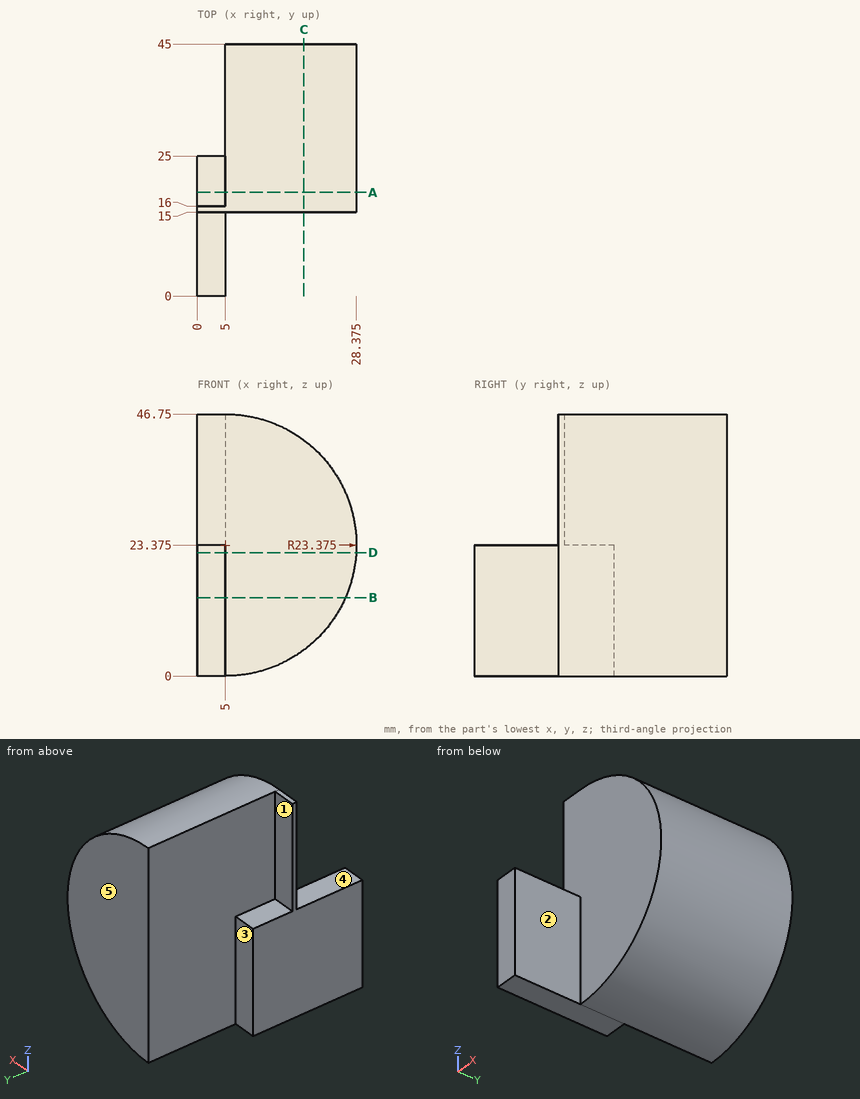
Design review of the part shown in the three views and the two pictorial views. Dimensions are in mm from the part's minimum x, y and z. A direction names the side the tool comes from. Round coordinates to 2 decimals unless told otherwise and drop trailing zeros. Loops run counter-clockwise (first coordinate to the right, second up) from the corner with the lowest first, then second, coordinate; pieces in that order, holes last.
1) Tool access review of the marked faces 1, 2, 3, 4 and 5: name each direction out of +Z, -Z, +X, -X, +Y, -Y from which nothing blocks a thin tool from reaching the whole face with its end or side.
Values follow:
face 1: +Z, -X, +Y
face 2: +Z, -Z, +X, -Y
face 3: +Z, -Z, -X, +Y
face 4: +Z, +X, -X, -Y
face 5: +Z, -Z, +X, -X, +Y
2) Consider section D-D on z = 22. State the section outline as (x, y) points, then the cut area to 3 significant figures.
Values follow:
outline: (0, 0) - (5, 0) - (5, 15) - (28.33, 15) - (28.33, 45) - (5, 45) - (5, 25) - (0, 25) - close
area: 825 mm2
3) Wall thickness on line 1 along Y through (x, z) = (24.25, 22.5); line 2 along X through (y, z) = (12, 20); line 3 along X through (y, z) = (27, 23): over which ranges is each line inside the solid? List them lowest first.
Values follow:
line 1: y = 15 to 45
line 2: x = 0 to 5
line 3: x = 5 to 28.37
4) Clearance check with flat-ended pins moving along their axes: P1, Ø1, axis at x = 4, z = 12.5, coming from the +Y side; P2, Ø2.5, axis at x = 2.5, y = 20.5, coming from the +Z side (3 decimals); P3, Ø6, axis at y = 22, z = 7, coming from the +X side. State where each tip first meets the part, or that it passes through.
Values follow:
P1: stops at y = 25
P2: stops at z = 23.375
P3: stops at x = 24.17
5) Consider section A-A on y = 18.5. State the section outline as (x, z) points (3 decimals), then the cut area to 3 significant figures.
Values follow:
outline: (0, 0) - (5, 0) arc R23.375 ccw to (5, 46.75) - (5, 23.375) - (0, 23.375) - close
area: 975 mm2
6) Consider section B-B on z = 14. State the section outline as (x, y) points.
Values follow:
outline: (0, 0) - (5, 0) - (5, 15) - (26.41, 15) - (26.41, 45) - (5, 45) - (5, 25) - (0, 25) - close
7) Consider section C-C on x = 19. State the section outline as (y, z) points, then the cut area to 3 significant figures.
Values follow:
outline: (15, 4.66) - (45, 4.66) - (45, 42.09) - (15, 42.09) - close
area: 1,120 mm2
